For this review, take the finished solid that the model builds, in its own axes (mm). Face numbers are marked on the shaded views. A direction names the side the tool comes from. Coordinates: 2 decimals unless noted, no trailing zeros. Write each loop counter-clockwise with the first axis right and the second up, starting at its lowest first coordinate (ties: lowest second). Pieces come first, ordered by that corner, then holes. Notation, with made-up numbers: (18, 36) - (27, 36) arc R15 ccw to (27, 41) - close; hole circle Ø2 at (3, 81.5). An arc over 180 degrees is marked (long way). Write each question's results on one line, items separated by ' | '.
from build123d import *

# Parameters (mm, degrees)
F0_W     = 76.2
F0_H     = 76.2
F1_DEPTH = 38.1
F2_R     = 11.1125
F3_DEPTH = 38.101
F6_DEPTH = 20.6375
F4_W     = 44.45
F4_H     = 25.4
F7_DEPTH = 76.201
F9_DEPTH = 76.201


with BuildPart() as f1:
    # F0 (on Front) → F1 (new body, symmetric)
    with BuildSketch(Plane.XZ):
        Rectangle(F0_W, F0_H)
    extrude(amount=F1_DEPTH, both=True)

    # F2 (on Front) → F3 (cut, through all)
    with BuildSketch(Plane.XZ):
        Circle(F2_R)
    extrude(amount=F3_DEPTH, mode=Mode.SUBTRACT)

    # F5 (on Right) → F6 (cut, symmetric)
    with BuildSketch(Plane.YZ):
        Polygon((-38.1, 19.05), (-27.101477, 38.1), (-38.1, 38.1), align=None)
    extrude(amount=F6_DEPTH, both=True, mode=Mode.SUBTRACT)

    # F4 (on face) → F7 (cut, through all)
    with BuildSketch(Plane.XY.offset(38.1)):
        with Locations((15.875, 25.4)):
            Rectangle(F4_W, F4_H)
    extrude(amount=-F7_DEPTH, mode=Mode.SUBTRACT)

    # F8 (on face) → F9 (cut, through all)
    with BuildSketch(Plane(origin=(-38.1, 0, 0), x_dir=(0, -1, 0), z_dir=(-1, 0, 0))):
        Polygon((22.225, -24.079956), (-3.175, -33.3248), (22.225, -33.3248), align=None)
    extrude(amount=-F9_DEPTH, mode=Mode.SUBTRACT)


solid = f1.part
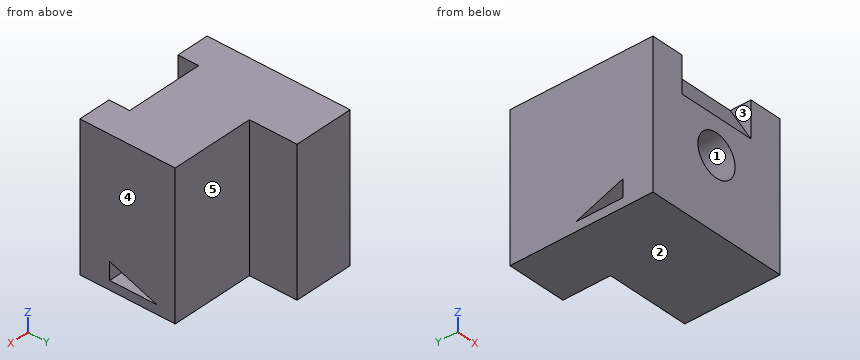
Q1. For the marked faces 1, 2, 3, 4 and 5, list the 3-axis set-ups (+Z, -Z, +X, -X, +Y, -Y) from which the entire face can be reached by the end or side of a thin tool; tool diameter is ignored.
Results found:
face 1: -Y | face 2: -Z, +X, -X, +Y, -Y | face 3: +Z, -Y | face 4: +Z, -Z, +X, +Y, -Y | face 5: +Z, -Z, +X, +Y
Q2. Take a section at A-A on x = 13. State the section outline as (y, z) points (3 decimals).
Results found:
outline: (-38.1, -38.1) - (12.7, -38.1) - (12.7, 38.1) - (-27.101, 38.1) - (-38.1, 19.05) - close; hole (-22.225, -33.325) - (3.175, -33.325) - (-22.225, -24.08) - close
Q3. For pin 1 (4 mm diameter, centred on y = 15, z = 19.5, fed in from +X); pin 2 (13.5 mm diameter, centred on x = 15, z = -5.5, fed in from +Y); pin 3 (20 mm diameter, centred on x = 0, z = 0, fed in from -Y); pin 4 (7.5 mm diameter, centred on x = -3.5, z = -30.5, fed in from +Y), all flat-tipped, find the tip position at first contact; note any pin that passes through.
Results found:
pin 1: x = -6.35 | pin 2: y = 12.7 | pin 3: y = 0 | pin 4: y = 38.1
Q4. Take a section at D-D on z = -21.5. State the section outline as (x, y) points, plus the area to 3 significant figures.
Results found:
outline: (-38.1, -38.1) - (38.1, -38.1) - (38.1, 12.7) - (-6.35, 12.7) - (-6.35, 38.1) - (-38.1, 38.1) - close | area: 4,680 mm2
Q5. Take a section at C-C on y = -24. State the section outline as (x, z) points (1 decimal).
Results found:
outline: (-38.1, -38.1) - (38.1, -38.1) - (38.1, 38.1) - (-38.1, 38.1) - close; hole circle Ø22.2 at (0, 0)
Q6. Take a section at B-B on y = -8. State the section outline as (x, z) points (1 decimal), plus the area to 3 significant figures.
Results found:
outline: (-38.1, -38.1) - (38.1, -38.1) - (38.1, -33.3) - (-38.1, -33.3) - close; (-38.1, -29.3) - (38.1, -29.3) - (38.1, 38.1) - (-38.1, 38.1) - close; hole circle Ø22.2 at (0, 0) | area: 5,110 mm2
Q7. Wall thickness on line 1 along X through (y, z) = (-8, 0); line 2 along Z through (x, y) = (0, -10.5); line 3 along Z through (x, y) = (0, -16.5): over which ranges is each line inside the solid? List them lowest first. Write a range as from..to.
Results found:
line 1: -38.1..-11.11, 11.11..38.1 | line 2: -38.1..-33.32, -28.35..-11.11, 11.11..38.1 | line 3: -38.1..-33.32, -26.16..-11.11, 11.11..38.1
